from build123d import *

# Parameters (mm, degrees)
F0_W     = 10.16
F0_H     = 14.0335
F1_DEPTH = 3.175
F0_H_2   = 5.08
F0_H_3   = 1.524
F2_DEPTH = 4.7625
F3_R     = 1.27


with BuildPart() as f1:
    # F0 (on Top) → F1 (new body)
    with BuildSketch(Plane.XY):
        with Locations((0, 1.778)):
            Rectangle(F0_W, F0_H)
    extrude(amount=F1_DEPTH)

    # F0 (on Top) → F2 (join)
    with BuildSketch(Plane.XY):
        with Locations((0, -7.77875)):
            Rectangle(F0_W, F0_H_2)
        with Locations((0, 9.55675)):
            Rectangle(F0_W, F0_H_3)
    extrude(amount=F2_DEPTH)

    # F3
    f3_edges = [f1.edges().sort_by_distance(p)[0] for p in [
        (0, -5.23875, 4.7625),
    ]]
    fillet(f3_edges, radius=F3_R)


solid = f1.part
Design review of the part built by this model. Coordinates are the model's own, in mm. A direction names the side the tool comes from. Coordinates: 2 decimals unless noted, no trailing zeros. Loops run counter-clockwise (first coordinate to the right, second up) from the corner with the lowest first, then second, coordinate; pieces in that order, holes last. Notation, with made-up numbers: (-31, -16.5) -> (-22, -16.5) arc R21 ccw to (-22, 21.5) -> close; hole circle Ø5 at (-16, 82.25). An arc over 180 degrees is marked (long way). Use a Markdown table: item, result. Add a question column.
Item 1: Wall thickness on L1, parallel to Y at x = -0.25, z = 3.4; L2, parallel to Z at x = 0, y = 5.5 (3 decimals); L3, parallel to Y at x = -3, z = 4.25: over which ranges is each line inside the solid? List them lowest first. Write a range as from..to.
Item 2: We need section B-B, the plane z = 4.3. Write out the cut boundary in (x, y), and give its area (3 significant figures).
Item 3: Machinability: for faces 1 (the flat face through (0, 10, 4.762)), 2 (the flat face through (0, 8.795, 4)), which of the approach directions +Z, -Z, +X, -X, +Y, -Y give a long, thin tool a straight path to every point of the face, cutting with its end or side? Answer none if there is none.
Item 4: We need section C-C, the plane y = -4. Write out the cut boundary in (x, z) (3 decimals), and give its area (3 significant figures).
Item 5: The part is to be moulded in two halves that separate along Y. For faces 3 (the flat face through (0, -8, 4.762)), 4 (the flat face through (0, 2, 3.175)), 5 (the flat face through (0, -10.319, 2)), 6 (the flat face through (0, 10.319, 2)), say which applies: +Y half, -Y half, draft (parallel to the pull), parting line (faces both ways), or undercut.
Item 6: Clearance check with flat-ended pins moving along their axes: P1, Ø3, axis at x = -0.5, y = 0.5, coming from the +Z side (3 decimals); P2, Ø6, axis at x = -0.5, y = 8, coming from the -Z side. State where each tip first meets the part, or that it passes through.
Numbers:
| question | item | result |
|---|---|---|
| 1 | L1 | y = -10.32..-5.24, 8.79..10.32 |
| 1 | L2 | z = 0..3.175 |
| 1 | L3 | y = -10.32..-5.49, 8.79..10.32 |
| 2 | outline | (-5.08, -10.32) -> (5.08, -10.32) -> (5.08, -5.53) -> (-5.08, -5.53) -> close; (-5.08, 8.79) -> (5.08, 8.79) -> (5.08, 10.32) -> (-5.08, 10.32) -> close |
| 2 | area | 64.2 mm^2 |
| 3 | face 1 | +Z, +X, -X, +Y, -Y |
| 3 | face 2 | +Z, +X, -X |
| 4 | outline | (-5.08, 0) -> (5.08, 0) -> (5.08, 3.175) -> (-5.08, 3.175) -> close |
| 4 | area | 32.3 mm^2 |
| 5 | face 3 | draft |
| 5 | face 4 | undercut |
| 5 | face 5 | -Y half |
| 5 | face 6 | +Y half |
| 6 | P1 | stops at z = 3.175 |
| 6 | P2 | stops at z = 0 |
